Autodesk Inventor part; units mm, degrees
ref_plane "YZ Plane" through (0, 0, 0) normal (1, 0, 0) x (0, 1, 0)
ref_plane "XZ Plane" through (0, 0, 0) normal (0, 1, 0) x (-1, 0, 0)
ref_plane "XY Plane" through (0, 0, 0) normal (0, 0, 1) x (1, 0, 0)
sketch "Sketch5" plane through (0, 0, 0) normal (0, 0, 1) x (1, 0, 0)
  line L0 (52.5, -14.7318) -> (52.5, -9.0024)
  line L1 (52.5, -9.0024) -> (50, -9.0024)
  line L2 (50, -9.0024) -> (50, -11.0274)
  line L3 (44, -11.0274) -> (44, -1.3774)
  line L4 (50, -1.3774) -> (50, -3.4024)
  line L5 (50, -3.4024) -> (52.5, -3.4024)
  line L6 (52.5, -3.4024) -> (52.5, 2.327)
  line L7 (44, -1.3774) -> (50, -1.3774)
  line L8 (44, -11.0274) -> (50, -11.0274)
  line L9 (52.5, -14.7318) -> (44, -14.7318)
  line L10 (40.2429, -14.7318) -> (44, -14.7318)
  line L11 (0, -14.7318) -> (40.2429, -14.7318)
  line L12 (0, -14.7318) -> (0, -2.8824)
  line L13 (0, -2.8824) -> (29.5442, 2.327)
  line L14 (29.5442, 2.327) -> (52.5, 2.327)
  point P0 (0, 0)
  dimension "d41" = 6
  dimension "d48" = 44
  dimension "d50" = 2.5
  dimension "d87" = 5.6
  dimension "d88" = 9.65
  dimension "d115" = 10
  dimension "d116" = 30
  dimension "d117" = 0
extrude "Extrusion2" add sketch "Sketch5" along normal blind 12
sketch "Sketch11" plane through (0, 0, 12) normal (0, 0, 1) x (1, 0, 0)
  line L0 (44, -1.3774) -> (50, -1.3774)
  circle A0 centre (44, -1.3774) radius 0.5
  line L1 (44, -11.0274) -> (44, -1.3774)
  circle A1 centre (44, -11.0274) radius 0.5
  line L2 (50, -11.0274) -> (44, -11.0274)
  circle A2 centre (50, -11.0274) radius 0.5
  line L3 (50, -1.3774) -> (50, -3.4024)
  circle A3 centre (50, -1.3774) radius 0.5
  point P0 (0, 0)
  dimension "d99" = 1
  dimension "d100" = 1
  dimension "d101" = 1
  dimension "d102" = 1
extrude "Extrusion7" cut sketch "Sketch11" against normal through all
fillet "Rundung4" radius 8 1 edges at (0, -14.7318, 6)
equation "\"l1\" = 8"
properties part number "Maria_Greifer_Dreieck2_3D-Druck"
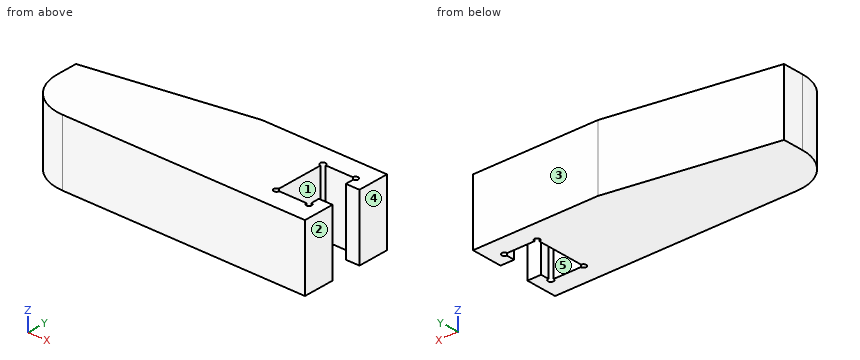
Verification items for the finished model (mm, model axes). Face numbers are marked on the shaded views. A direction names the side the tool comes from. Coordinates: 2 decimals unless noted, no trailing zeros. Loops run counter-clockwise (first coordinate to the right, second up) from the corner with the lowest first, then second, coordinate; pieces in that order, holes last. Notation, with made-up numbers: (78.25, 24.25) - (102.25, 24.25) arc R32 ccw to (102.25, 55.25) - close; hole circle Ø2 at (28.5, 50.25). An arc over 180 degrees is marked (long way). Answer as a JSON object with one key per item and string values.
(1) Scan lines: line 1 along X through (y, z) = (-3, 8.75); line 2 along X through (y, z) = (-5.5, 0.5); line 3 along Y through (x, z) = (4, 4.25). Record each from-to range of solid material in increasing order.
Response:
{"line 1": "x = 0 to 44, 50 to 52.5", "line 2": "x = 0 to 44", "line 3": "y = -13.66 to -2.18"}
(2) Access from +Z, -Z, +X, -X, +Y, -Y to the whole of each face (thin tool, end or side, straight path). Record for the marked faces 1 and 2.
Response:
{"face 1": "+Z, -Z", "face 2": "+Z, -Z, +X, +Y, -Y"}
(3) Go/stop test with flat-tipped pins: pin 1 Ø7 at (y, z) = (-5.5, 8.5) entering from +X; pin 2 Ø1.7 at (y, z) = (-9.5, 5.5) entering from -X; pin 3 Ø1.5 at (x, z) = (27.5, 8.5) entering from +Y. Record where each tip stops, or that it passes through.
Response:
{"pin 1": "stops at x = 52.5", "pin 2": "stops at x = 0.23", "pin 3": "stops at y = 2.1"}
(4) Cross-section at B-B, the plane z = 2.5. Record the boundary of the cut face in (x, y), then the cut area to 3 significant figures.
Response:
{"outline": "(0, -6.73) arc R8 ccw to (8, -14.73) - (52.5, -14.73) - (52.5, -9) - (50, -9) - (50, -10.53) arc R0.5 cw (long way) to (49.5, -11.03) - (44.5, -11.03) arc R0.5 cw (long way) to (44, -10.53) - (44, -1.88) arc R0.5 cw (long way) to (44.5, -1.38) - (49.5, -1.38) arc R0.5 cw (long way) to (50, -1.88) - (50, -3.4) - (52.5, -3.4) - (52.5, 2.33) - (29.54, 2.33) - (0, -2.88) - close", "area": "731 mm²"}
(5) Cross-section at A-A, the plane y = -10. Record the boundary of the cut face in (x, z).
Response:
{"outline": "(0.7, 0) - (44, 0) - (44, 12) - (0.7, 12) - close; (50, 0) - (52.5, 0) - (52.5, 12) - (50, 12) - close"}
(6) Mould release check, pull along X, two halves, no side actions. Record for the marked faces 3, 4 and 5: pulls with the +X half, pulls with the -X half, needs draft (parallel to the pull), parting line crosses it, or undercut.
Response:
{"face 3": "needs draft", "face 4": "pulls with the +X half", "face 5": "undercut"}
(7) Cross-section at D-D, the plane x = 20. Record the boundary of the cut face in (y, z).
Response:
{"outline": "(-14.73, 0) - (0.64, 0) - (0.64, 12) - (-14.73, 12) - close"}
(8) Cross-section at C-C, the plane y = -5.5. Record the boundary of the cut face in (x, z).
Response:
{"outline": "(0, 0) - (44, 0) - (44, 12) - (0, 12) - close"}
